from build123d import *

# Parameters (mm, degrees)
EXTRUDE_1_DEPTH             = 126
CHAMFER_1_SIZE              = 11
HOLE_WIZARD_M51_D           = 5.8
HOLE_WIZARD_M51_DEPTH       = 3
HOLE_WIZARD_M51_CSINK_D     = 6
HOLE_WIZARD_M51_CSINK_ANGLE = 90
HOLE_WIZARD_M51_TIP         = 1.742495795
HOLE_WIZARD_M52_D           = 5.8
HOLE_WIZARD_M52_DEPTH       = 3
HOLE_WIZARD_M52_CSINK_D     = 6
HOLE_WIZARD_M52_CSINK_ANGLE = 90
HOLE_WIZARD_M52_TIP         = 1.742495795


with BuildPart() as part:
    # Эскиз1 → Бобышка-Вытянуть1 (new body)
    with BuildSketch(Plane.XY):
        Polygon((0, 0), (0, 15), (2, 15), (2, 2), (15, 2), (15, 0), align=None)
    extrude(amount=EXTRUDE_1_DEPTH)

    # Фаска1
    chamfer_1_edges = [part.edges().sort_by_distance(p)[0] for p in [
        (1, 15, 126),
        (1, 15, 0),
        (15, 1, 126),
        (15, 1, 0),
    ]]
    chamfer(chamfer_1_edges, length=CHAMFER_1_SIZE)

    # Эскиз2 → Зенковка для винта с потайной головкой M41 (revolve, cut)
    with BuildSketch(Plane(origin=(7, 0, 116), x_dir=(0, 0, -1), z_dir=(1, 0, 0))):
        Polygon((0, 0), (0, 2), (2.4, 2), (2.25, 1.85), (2.25, 1.45), (3.7, 0), align=None)
    revolve(axis=Axis((7, -6.35, 116), (0, 1, 0)), mode=Mode.SUBTRACT)

    # Эскиз4 → Зенковка для винта с потайной головкой M42 (revolve, cut)
    with BuildSketch(Plane(origin=(0, 7, 10), x_dir=(0, 0, 1), z_dir=(0, 1, 0))):
        Polygon((0, 0), (0, 2), (2.4, 2), (2.25, 1.85), (2.25, 1.45), (3.7, 0), align=None)
    revolve(axis=Axis((-6.35, 7, 10), (1, 0, 0)), mode=Mode.SUBTRACT)

    # Отверстие с зазором M51
    with Locations(Plane.XZ):
        with Locations((8, 59)):
            CounterSinkHole(HOLE_WIZARD_M51_D / 2, HOLE_WIZARD_M51_CSINK_D / 2, depth=HOLE_WIZARD_M51_DEPTH, counter_sink_angle=HOLE_WIZARD_M51_CSINK_ANGLE)
            with Locations((0, 0, -(HOLE_WIZARD_M51_DEPTH + HOLE_WIZARD_M51_TIP / 2))):  # 118° drill point
                Cone(0, HOLE_WIZARD_M51_D / 2, HOLE_WIZARD_M51_TIP, mode=Mode.SUBTRACT)

    # Отверстие с зазором M52
    with Locations(Plane.ZY):
        with Locations((67, 8)):
            CounterSinkHole(HOLE_WIZARD_M52_D / 2, HOLE_WIZARD_M52_CSINK_D / 2, depth=HOLE_WIZARD_M52_DEPTH, counter_sink_angle=HOLE_WIZARD_M52_CSINK_ANGLE)
            with Locations((0, 0, -(HOLE_WIZARD_M52_DEPTH + HOLE_WIZARD_M52_TIP / 2))):  # 118° drill point
                Cone(0, HOLE_WIZARD_M52_D / 2, HOLE_WIZARD_M52_TIP, mode=Mode.SUBTRACT)


solid = part.part
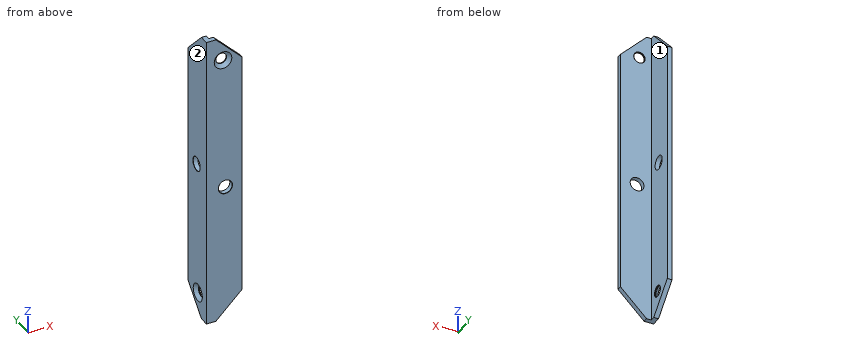
Can you work these out from the model? Positions are in its coordinate system, mm. Face numbers are marked on the shaded views. A direction names the side the tool comes from. Give positions to 0.01 mm unless a question says otherwise; leave off trailing zeros. Order: outer loops, then holes, each group sorted by start corner. A loop starts at its lowest first (then second) coordinate and runs counter-clockwise, first axis right, second up. Notation, with made-up numbers: M 51,5.5 L 68,5.5 A20 cw 68,12.5 Z; hole C 73.5,8.25 d8. An arc over 180 degrees is marked long. Use one line per item in the form item = value.
Item 1: For the marked faces 1 and 2, which set-ups out of +Z, -Z, +X, -X, +Y, -Y let a thin tool reach every point of the face, with its end or its side?
Values follow:
face_1 = +Z, -Z, +X, +Y
face_2 = +Z, -Z, -X, +Y, -Y
Item 2: If we section it at A-A, the plane z = 67: Write out the boundary of the cut face in (x, y), and give its area (3 significant figures).
Values follow:
outline = M 0,0 L 15,0 L 15,2 L 2,2 L 2,5.1 L 0.1,5.1 L 0,5 Z; M 0,11 L 0.1,10.9 L 2,10.9 L 2,15 L 0,15 Z
area = 44.4 mm^2
Item 3: If we section it at D-D, the plane x = 13: Write out the boundary of the cut face in (y, z), and give its area (3 significant figures).
Values follow:
outline = M 0,9 L 2,9 L 2,117 L 0,117 Z
area = 216 mm^2
Item 4: Will these pins go through, and if not, where does the flat tip stop? pin 1 Ø2 at (x, z) = (6, 18) entering from -Y; pin 2 Ø7 at (y, z) = (7, 10) entering from +X; pin 3 Ø6 at (x, z) = (7, 116) entering from +Y; pin 4 Ø4 at (x, y) = (3.5, 8) entering from +Z.
Values follow:
pin_1 = 0
pin_2 = 2
pin_3 = 2
pin_4 = 123.32
Item 5: If I drill on line 1 along Z through (x, y) = (8, 0.55); line 2 along X through (y, z) = (7.25, 42.5); line 3 along Z through (x, y) = (1.6, 7), over which ranges is the centre line in solid material (lowest first)? Write a range as [from, to].
Values follow:
line_1 = [4, 56.1], [61.9, 113.01], [118.99, 122]
line_2 = [0, 2]
line_3 = [3, 7.75], [12.25, 64.28], [69.72, 123]
Item 6: If we section it at B-B, the plane z = 39: Write out the boundary of the cut face in (x, y), and give its area (3 significant figures).
Values follow:
outline = M 0,0 L 15,0 L 15,2 L 2,2 L 2,15 L 0,15 Z
area = 56.0 mm^2
Item 7: If we section it at C-C, the plane x = 7: Count the separate pieces of the cut face and the enclosed holes in it, and give its area (3 significant figures).
Values follow:
separate_pieces = 3
enclosed_holes = 0
area = 218 mm^2
